Input: dimensioned drawing with shaded views. Units: mm. Origin: part minimum x, y, z. A direction names the side the tool comes from. Round coordinates to 2 decimals unless told otherwise and drop trailing zeros. Order: outer loops, then holes, each group sorted by start corner. A loop starts at its lowest first (then second) coordinate and runs counter-clockwise, first axis right, second up. Notation, with made-up numbers: (51, -17) - (88, -17) arc R28 ccw to (88, 11) - close; hole circle Ø6 at (23.5, -5). An arc over 180 degrees is marked (long way). Return JSON: item names as keys, results as strings. Group by question number.
1) Section B-B, the plane y = 13. Return loops of the section in (x, z).
2) Section A-A, the plane x = 24.13. Return loops of the section in (y, z) (1 decimal).
3) Ray query, line 1 (Z direction, x = 15.24, y = 1.65) (1 decimal); line 2 (Z direction, x = 6.35, y = 1) (1 decimal); line 3 (Z direction, x = 15.24, y = 4) (1 decimal). Return the intervals inside material, ascending. Write a range as from..to.
4) Mould query, pull axis X, two halves, no side actions, for the marked faces 1, 2, 3 and 4. Classes: pulls with the +X half, pulls with the -X half, needs draft (parallel to the pull), parting line crosses it, or undercut.
5) Section C-C, the plane z = 6.35. Return loops of the section in (x, y) (1 decimal).
6) Access query for the marked faces 5, 6 and 7. Directions: +Z, -Z, +X, -X, +Y, -Y. A direction counts if a zero-diameter tool reaches every point of the face in a straight line with its end or side. Return the directions, or none.
7) Contact query for flat-ended pins moving along their axis: P1, Ø3, axis at x = 21.5, y = 15.5, coming from the -Z side; P2, Ø5, axis at x = 9, y = 11.5, coming from the +Z side; P3, Ø8, axis at x = 14.5, z = 8, coming from the +Y side; P4, Ø1.5, axis at x = 14, z = 56.5, coming from the +Y side. Output: stop coordinate, or through.
8) Section D-D, the plane y = 1.5. Give the number of separate pieces and of enclosed holes in the cut face, plus the area to 3 significant figures.
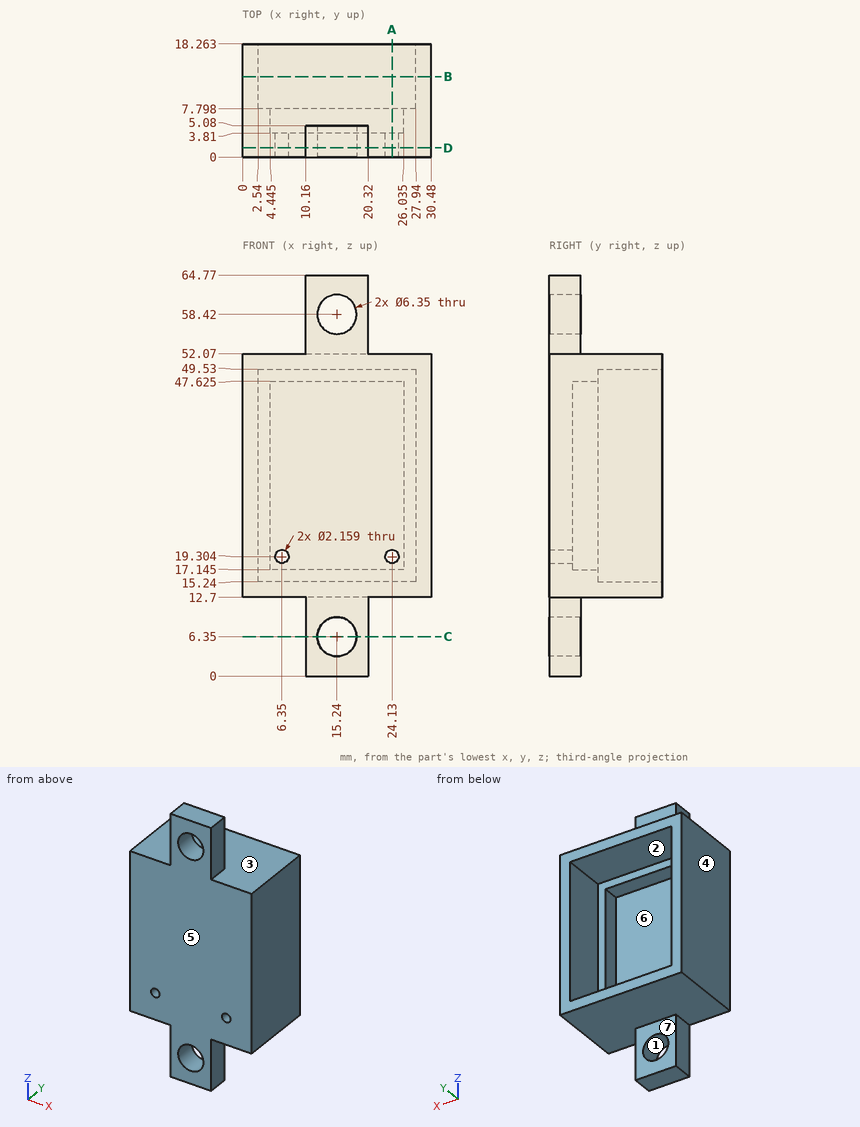
Geometry check:
{
 "1": {"outline": "(0, 12.7) - (30.48, 12.7) - (30.48, 52.07) - (0, 52.07) - close; hole (2.54, 15.24) - (27.94, 15.24) - (27.94, 49.53) - (2.54, 49.53) - close"},
 "2": {"outline": "(0, 12.7) - (18.3, 12.7) - (18.3, 15.2) - (7.8, 15.2) - (7.8, 17.1) - (3.8, 17.1) - (3.8, 18.2) - (0, 18.2) - close; (0, 20.4) - (3.8, 20.4) - (3.8, 47.6) - (7.8, 47.6) - (7.8, 49.5) - (18.3, 49.5) - (18.3, 52.1) - (0, 52.1) - close"},
 "3": {"line 1": "0..3.2, 9.5..55.2, 61.6..64.8", "line 2": "12.7..18.2, 20.4..52.1", "line 3": "0..3.2, 9.5..17.1, 47.6..55.2, 61.6..64.8"},
 "4": {"face 1": "undercut", "face 2": "undercut", "face 3": "needs draft", "face 4": "pulls with the -X half"},
 "5": {"outline": "(10.2, 0) - (12.1, 0) - (12.1, 5.1) - (10.2, 5.1) - close; (18.4, 0) - (20.3, 0) - (20.3, 5.1) - (18.4, 5.1) - close"},
 "6": {"face 5": "+Z, -Z, +X, -X, -Y", "face 6": "+Y", "face 7": "-Z, +X, -X, +Y"},
 "7": {"P1": "z = 12.7", "P2": "z = 52.07", "P3": "y = 5.08", "P4": "through"},
 "8": {"separate pieces": "1", "enclosed holes": "4", "area": "1,390 mm2"}
}
